from build123d import *

# Parameters (mm, degrees)
SKETCH_1_W                = 12
SKETCH_1_H                = 19
EXTRUDE_1_REACH           = 37.781
EXTRUDE_1_END_RADIUS      = 12
SKETCH_2_W                = 14
SKETCH_2_H                = 16
EXTRUDE_2_REACH           = 34.679
EXTRUDE_2_START_RADIUS    = 12
EXTRUDE_2_END_RADIUS      = 12
SKETCH_3_W                = 1
SKETCH_3_H                = 7
EXTRUDE_3_REACH           = 34.679
EXTRUDE_3_START_RADIUS    = 12
EXTRUDE_3_END_RADIUS      = 12
SKETCH_4_W                = 1
SKETCH_4_H                = 7
SKETCH_5_W                = 2.5
SKETCH_5_H                = 5
HOLE_WIZARD_4_0_4_1_D     = 4
HOLE_WIZARD_4_0_4_1_DEPTH = 19
CHAMFER_1_SIZE            = 1


with BuildPart() as part:
    # 草图1 → 旋转1 (revolve)
    with BuildSketch(Plane.XZ, mode=Mode.PRIVATE) as revolve_1_sk:
        with Locations((6, -8.5)):
            Rectangle(SKETCH_1_W, SKETCH_1_H)
    revolve(revolve_1_sk.sketch.rotate(Axis((0, 0, 1), (0, 0, -1)), 180), axis=Axis((0, 0, 1), (0, 0, -1)))

    # 凸台-拉伸1: up to this cylinder (the profile starts outside it)
    extrude_1_end = Plane(origin=(0, 0, -7), z_dir=(0, 0, -1)) * Cylinder(EXTRUDE_1_END_RADIUS, 100.562, mode=Mode.PRIVATE)
    # 草图2 → 凸台-拉伸1 (add, up to the surface)
    with BuildSketch(Plane(origin=(0, 16.5, 0), x_dir=(1, 0, 0), z_dir=(0, 1, 0)), mode=Mode.PRIVATE) as extrude_1_sk1:
        with Locations((0, 7)):
            Rectangle(SKETCH_2_W, SKETCH_2_H)
    extrude_1_tool1 = extrude(extrude_1_sk1.sketch, amount=-EXTRUDE_1_REACH, mode=Mode.PRIVATE) - extrude_1_end
    add(extrude_1_tool1.solids().sort_by_distance((0, 16.5, -7))[0])

    # 凸台-拉伸2: from a cylinder face, 34.679 long prism both ways, kept between that surface and its translate by the depth
    extrude_2_start = Plane(origin=(0, 0, 0.5), z_dir=(0, 0, -1)) * Cylinder(EXTRUDE_2_START_RADIUS, 94.358, mode=Mode.PRIVATE)
    extrude_2_end = Plane(origin=(4.021759717, 0, 0.5), z_dir=(0, 0, -1)) * Cylinder(EXTRUDE_2_END_RADIUS, 94.358, mode=Mode.PRIVATE)
    # 草图3 → 凸台-拉伸2 (add, from a surface)
    with BuildSketch(Plane(origin=(-3, 0, 0), x_dir=(0, 0, -1), z_dir=(1, 0, 0)), mode=Mode.PRIVATE) as extrude_2_sk1:
        with Locations((-0.5, 0)):
            Rectangle(SKETCH_3_W, SKETCH_3_H)
    extrude_2_tool1 = extrude(extrude_2_sk1.sketch, amount=EXTRUDE_2_REACH, both=True, mode=Mode.PRIVATE)
    add(((extrude_2_tool1 - extrude_2_start) & extrude_2_end).solids().sort_by_distance((13.48912, 0, 0.5))[0])

    # 凸台-拉伸3: from a cylinder face, 34.679 long prism both ways, kept between that surface and its translate by the depth
    extrude_3_start = Plane(origin=(0, 0, 0.5), z_dir=(0, 0, -1)) * Cylinder(EXTRUDE_3_START_RADIUS, 94.358, mode=Mode.PRIVATE)
    extrude_3_end = Plane(origin=(-4.021759717, 0, 0.5), z_dir=(0, 0, -1)) * Cylinder(EXTRUDE_3_END_RADIUS, 94.358, mode=Mode.PRIVATE)
    # 草图4 → 凸台-拉伸3 (add, from a surface)
    with BuildSketch(Plane.ZY.offset(-3), mode=Mode.PRIVATE) as extrude_3_sk1:
        with Locations((0.5, 0)):
            Rectangle(SKETCH_4_W, SKETCH_4_H)
    extrude_3_tool1 = extrude(extrude_3_sk1.sketch, amount=EXTRUDE_3_REACH, both=True, mode=Mode.PRIVATE)
    add(((extrude_3_tool1 - extrude_3_start) & extrude_3_end).solids().sort_by_distance((-13.48912, 0, 0.5))[0])

    # 草图5 → 旋转2 (revolve)
    with BuildSketch(Plane.XZ.offset(6.5), mode=Mode.PRIVATE) as revolve_2_sk:
        with Locations((1.25, 3.5)):
            Rectangle(SKETCH_5_W, SKETCH_5_H)
    revolve(revolve_2_sk.sketch.rotate(Axis((0, -6.5, 6), (0, 0, -1)), 180), axis=Axis((0, -6.5, 6), (0, 0, -1)))

    # Ø4.0 (4) 直径孔1
    with Locations(Plane.XY.offset(1)):
        with Locations((-15.5, 0), (15.5, 0)):
            Hole(HOLE_WIZARD_4_0_4_1_D / 2, depth=HOLE_WIZARD_4_0_4_1_DEPTH)

    # 倒角1
    chamfer_1_edges = [part.edges().sort_by_distance(p)[0] for p in [
        (-7, 16.5, -7),
        (7, 16.5, -7),
    ]]
    chamfer(chamfer_1_edges, length=CHAMFER_1_SIZE)


solid = part.part
Here's how the part is built. I have some questions about the finished solid (model axes, mm). A direction names the side the tool comes from. Round coordinates to 2 decimals unless told otherwise and drop trailing zeros. Order: outer loops, then holes, each group sorted by start corner. A loop starts at its lowest first (then second) coordinate and runs counter-clockwise, first axis right, second up. Notation, with made-up numbers: (50, 66) -> (67, 66) arc R21 ccw to (67, 100) -> close; hole circle Ø11 at (-10.75, 18). An arc over 180 degrees is marked (long way). Use CSV: the item, a comma, the result in double quotes.
1. Which directions (+Z, -Z, +X, -X, +Y, -Y) give clear straight access to the entire face, cutting with the end or side of a thin tool? Please do faces 4 (the face through (13.5, -3.5, 0.5)), 5 (the face through (7, 13, -7)), 6 (the face through (-13.5, -3.5, 0.5)), 7 (the face through (-13.5, 3.5, 0.5)), 8 (the face through (0, -4, 4)).
Recorded:
face 4,"+Z, -Z, +X, -Y"
face 5,"+Z, -Z, +X, +Y"
face 6,"+Z, -Z, -X, -Y"
face 7,"+Z, -Z, -X, +Y"
face 8,"+Z"
2. I want a section at B-B on y = 0. List the corners of the cut face in (x, z) for me.
Recorded:
outline,"(-13.5, 0) -> (-12, 0) -> (-12, -18) -> (12, -18) -> (12, 0) -> (13.5, 0) -> (13.5, 1) -> (-13.5, 1) -> close"
3. I'm going to push flat-ended pins straight in: P1, Ø0.8, axis at x = -13, z = 0.5, coming from the +Y side; P2, Ø12, axis at y = 8, z = -4.5, coming from the -X side; P3, Ø8, axis at y = 9.5, z = -8.5, coming from the +X side. Where does each tip first touch, or does it pass through?
Recorded:
P1,"stops at y = 3.5"
P2,"stops at x = -11.83"
P3,"stops at x = 10.67"
4. I want a section at D-D on y = -8.25. List the corners of the cut face in (x, z) for me, and give its area (3 significant figures).
Recorded:
outline,"(-8.71, -18) -> (8.71, -18) -> (8.71, 1) -> (1.79, 1) -> (1.79, 6) -> (-1.79, 6) -> (-1.79, 1) -> (-8.71, 1) -> close"
area,"349 mm2"
5. I want a section at A-A on x = 0. List the corners of the cut face in (y, z) for me, and give its area (3 significant figures).
Recorded:
outline,"(-12, -18) -> (12, -18) -> (12, -15) -> (16.5, -15) -> (16.5, 1) -> (-4, 1) -> (-4, 6) -> (-9, 6) -> (-9, 1) -> (-12, 1) -> close"
area,"553 mm2"
6. I want a section at C-C on z = -0.5. List the corners of the cut face in (x, y) for me, and give its area (3 significant figures).
Recorded:
outline,"(-7, 9.75) arc R12 ccw (long way) to (7, 9.75) -> (7, 15.5) -> (6, 16.5) -> (-6, 16.5) -> (-7, 15.5) -> close"
area,"524 mm2"
7. I need wall thicknesses on line 1 along Z through (x, y) = (-6.5, -8); line 2 along X through (y, z) = (0, 0.25); line 3 along X through (y, z) = (15, -8.25). Which ranges of each line are inside material? Lowest first, please.
Recorded:
line 1,"z = -18 to 1"
line 2,"x = -13.5 to 13.5"
line 3,"x = -7 to 7"
8. Thinking about a two-plate mould opening in X: for faces 1 (the face through (2.601, -11.715, -8.367)), 2 (the face through (13.5, 0, 0.5)), 3 (the face through (0, 16.5, -7)), which applies, pulls with the +X half, pulls with the -X half, needs draft (parallel to the pull), parting line crosses it, or undercut?
Recorded:
face 1,"parting line crosses it"
face 2,"undercut"
face 3,"needs draft"
